from build123d import *

# Parameters (mm, degrees)
BOSS_EXTRUDE1_DEPTH = 18.14
FILLET1_R           = 1
SKETCH3_R           = 1
CUT_EXTRUDE1_DEPTH  = 5.1
SKETCH4_R           = 1
CUT_EXTRUDE2_DEPTH  = 5.1
SKETCH5_R           = 1.7
CUT_EXTRUDE3_DEPTH  = 1.4
SKETCH6_R           = 1.7
CUT_EXTRUDE4_DEPTH  = 1.4
LPATTERN1_COUNT     = 2
LPATTERN1_PITCH     = 6.52
LPATTERN2_COUNT     = 2
LPATTERN2_PITCH     = 6.52


with BuildPart() as part:
    # Sketch1 → Boss-Extrude1 (new body)
    with BuildSketch(Plane(origin=(0, 0, 0), x_dir=(1, 0, 0), z_dir=(0, 1, 0))):
        Polygon((0, 0), (0, 5.2), (-3, 5.2), (-3, -3), (5.2, -3), (5.2, 0), align=None)
    extrude(amount=BOSS_EXTRUDE1_DEPTH)

    # Fillet1
    fillet1_edges = [part.edges().sort_by_distance(p)[0] for p in [
        (-1.5, 18.14, -5.2),
        (5.2, 18.14, 1.5),
        (5.2, 0, 1.5),
        (-1.5, 0, -5.2),
    ]]
    fillet(fillet1_edges, radius=FILLET1_R)

    # Sketch3 → Cut-Extrude1 (cut)
    with BuildSketch(Plane(origin=(0, 0, 0), x_dir=(0, 0, -1), z_dir=(1, 0, 0))):
        with Locations((3, 15.59)):
            Circle(SKETCH3_R)
    cut_extrude1 = extrude(amount=-CUT_EXTRUDE1_DEPTH, mode=Mode.SUBTRACT)

    # Sketch4 → Cut-Extrude2 (cut)
    with BuildSketch(Plane(origin=(0, 0, 0), x_dir=(-1, 0, 0), z_dir=(0, 0, -1))):
        with Locations((-3, 2.55)):
            Circle(SKETCH4_R)
    cut_extrude2 = extrude(amount=-CUT_EXTRUDE2_DEPTH, mode=Mode.SUBTRACT)

    # Sketch5 → Cut-Extrude3 (cut)
    with BuildSketch(Plane(origin=(0, 0, 0), x_dir=(-1, 0, 0), z_dir=(0, 0, -1))):
        with Locations((-3, 2.55)):
            Circle(SKETCH5_R)
    cut_extrude3 = extrude(amount=-CUT_EXTRUDE3_DEPTH, mode=Mode.SUBTRACT)

    # Sketch6 → Cut-Extrude4 (cut)
    with BuildSketch(Plane.ZY.offset(3)):
        with Locations((-3, 15.59)):
            Circle(SKETCH6_R)
    cut_extrude4 = extrude(amount=-CUT_EXTRUDE4_DEPTH, mode=Mode.SUBTRACT)

    # Mirror2: Cut-Extrude1, Cut-Extrude2, Cut-Extrude3, Cut-Extrude4 across plane
    add(cut_extrude1.mirror(Plane.ZX.offset(9.07)), mode=Mode.SUBTRACT)
    add(cut_extrude2.mirror(Plane.ZX.offset(9.07)), mode=Mode.SUBTRACT)
    add(cut_extrude3.mirror(Plane.ZX.offset(9.07)), mode=Mode.SUBTRACT)
    add(cut_extrude4.mirror(Plane.ZX.offset(9.07)), mode=Mode.SUBTRACT)

    # LPattern1: Cut-Extrude1, Cut-Extrude4 ×2
    with Locations(*[(0, -i * LPATTERN1_PITCH, 0) for i in range(1, LPATTERN1_COUNT)]):
        add(cut_extrude1, mode=Mode.SUBTRACT)
        add(cut_extrude4, mode=Mode.SUBTRACT)

    # LPattern2: Cut-Extrude2, Cut-Extrude3 ×2
    with Locations(*[(0, i * LPATTERN2_PITCH, 0) for i in range(1, LPATTERN2_COUNT)]):
        add(cut_extrude2, mode=Mode.SUBTRACT)
        add(cut_extrude3, mode=Mode.SUBTRACT)


solid = part.part
Input: part model. Units: mm. Frame: model coordinates. A direction names the side the tool comes from. Give positions to 0.01 mm unless a question says otherwise; leave off trailing zeros. Loops run counter-clockwise (first coordinate to the right, second up) from the corner with the lowest first, then second, coordinate; pieces in that order, holes last. Notation, with made-up numbers: M -2,86 L 48,86 A5 cw 48,92 Z; hole C 15.5,7.25 d10. An arc over 180 degrees is marked long. Use one line per item in the form item = value.
1. First-contact query: pin 1 (1.6 mm diameter, centred on y = 15.59, z = -3, fed in from +X); pin 2 (1 mm diameter, centred on x = 3.5, y = 15, fed in from -Z); pin 3 (3 mm diameter, centred on y = 9.07, z = -3, fed in from -X); pin 4 (3.5 mm diameter, centred on x = 3.5, y = 2.5, fed in from -Z). Flat tips, straight axial feed; report the tip coordinate or a pass-through.
Numbers:
pin_1 = through
pin_2 = 1.4
pin_3 = -1.6
pin_4 = 0
2. Pull-direction query (Z, two-part tool) for faces 4 (the face through (-1.521, 0.301, -4.915)), 5 (the face through (-2.31, 14.08, -2.22)), 6 (the face through (0, 9, -1)), 7 (the face through (-0.79, 1.56, -2.87)); classes: released by +Z, released by -Z, zero draft, split by the parting line, or undercut.
Numbers:
face_4 = released by -Z
face_5 = undercut
face_6 = zero draft
face_7 = undercut
3. Section query C-C, the plane x = -1. Return the cut outline in (y, z), and give its area (3 significant figures).
Numbers:
outline = M 0,-4.2 A1 ccw 1,-5.2 L 17.14,-5.2 A1 ccw 18.14,-4.2 L 18.14,3 L 0,3 Z; hole C 2.55,-3 d2; hole C 9.07,-3 d2; hole C 15.59,-3 d2
area = 139 mm²
4. Line query: L1, parallel to Y at x = 3, z = 1.15; L2, parallel to Y at x = 3, z = 2; L3, parallel to X at y = 15.59, z = 0.55. Output: solid intervals per line, ascending.
Numbers:
L1 = 0 to 0.85, 4.25 to 7.37, 10.77 to 13.89, 17.29 to 18.14
L2 = 0 to 1.55, 3.55 to 8.07, 10.07 to 14.59, 16.59 to 18.14
L3 = -3 to 1.3, 4.7 to 5.2
5. Section query A-A, the plane x = 3. Return the cut outline in (y, z).
Numbers:
outline = M 0,0 L 0.85,0 L 0.85,1.4 L 1.55,1.4 L 1.55,3 L 0,3 Z; M 3.55,1.4 L 4.25,1.4 L 4.25,0 L 7.37,0 L 7.37,1.4 L 8.07,1.4 L 8.07,3 L 3.55,3 Z; M 10.07,1.4 L 10.77,1.4 L 10.77,0 L 13.89,0 L 13.89,1.4 L 14.59,1.4 L 14.59,3 L 10.07,3 Z; M 16.59,1.4 L 17.29,1.4 L 17.29,0 L 18.14,0 L 18.14,3 L 16.59,3 Z
6. Section query B-B, the plane z = -3. Return the cut outline in (x, y), and give its area (3 significant figures).
Numbers:
outline = M -3,0 L 0,0 L 0,1.55 L -1.6,1.55 L -1.6,0.85 L -3,0.85 Z; M -3,4.25 L -1.6,4.25 L -1.6,3.55 L 0,3.55 L 0,8.07 L -1.6,8.07 L -1.6,7.37 L -3,7.37 Z; M -3,10.77 L -1.6,10.77 L -1.6,10.07 L 0,10.07 L 0,14.59 L -1.6,14.59 L -1.6,13.89 L -3,13.89 Z; M -3,17.29 L -1.6,17.29 L -1.6,16.59 L 0,16.59 L 0,18.14 L -3,18.14 Z
area = 30.5 mm²
7. Section query D-D, the plane z = 2. Return the cut outline in (x, y), and give its area (3 significant figures).
Numbers:
outline = M -3,0 L 4.2,0 A1 ccw 5.2,1 L 5.2,17.14 A1 ccw 4.2,18.14 L -3,18.14 Z; hole C 3,2.55 d2; hole C 3,9.07 d2; hole C 3,15.59 d2
area = 139 mm²
8. Reachability of faces 1 (the face through (1.43, 16.24, 0.69)), 2 (the face through (-2.31, 8.42, -1.43)), 3 (the face through (3, 7, 0)) from +Z, -Z, +X, -X, +Y, -Y: full face, straight path, thin tool, end or side. Return the list, or none.
Numbers:
face_1 = -Z
face_2 = -X
face_3 = -Z, +X, +Y, -Y
